```python
from build123d import *

# Parameters (mm, degrees)
SKETCH_2_W           = 42
SKETCH_2_H           = 42
EXTRUDE_1_DEPTH      = 69
SKETCH_3_R           = 12.5
EXTRUDE_2_DEPTH      = 2
SKETCH_4_R           = 4.5
EXTRUDE_3_DEPTH      = 1
SKETCH_5_R           = 4
EXTRUDE_4_DEPTH      = 18
EXTRUDE_5_DEPTH      = 1.5
EXTRUDE_5_DEPTH_BACK = 4
SKETCH_7_R           = 1.75
CUT_EXTRUDE_1_DEPTH  = 71.5


with BuildPart() as part:
    # 草图2 → 凸台-拉伸1 (new body)
    with BuildSketch(Plane(origin=(0, 0, 0), x_dir=(1, 0, 0), z_dir=(0, 1, 0))):
        with Locations((21, 21)):
            Rectangle(SKETCH_2_W, SKETCH_2_H)
    extrude(amount=EXTRUDE_1_DEPTH)

    # 草图3 → 凸台-拉伸2 (add)
    with BuildSketch(Plane(origin=(0, 69, 0), x_dir=(1, 0, 0), z_dir=(0, 1, 0))):
        with Locations(Location((21, 21, 0), (0, 0, 270))):
            Circle(SKETCH_3_R)
    extrude(amount=EXTRUDE_2_DEPTH)

    # 草图4 → 凸台-拉伸3 (add)
    with BuildSketch(Plane(origin=(0, 71, 0), x_dir=(1, 0, 0), z_dir=(0, 1, 0))):
        with Locations(Location((21, 21, 0), (0, 0, 270))):
            Circle(SKETCH_4_R)
    extrude(amount=EXTRUDE_3_DEPTH)

    # 草图5 → 凸台-拉伸4 (add)
    with BuildSketch(Plane(origin=(0, 72, 0), x_dir=(1, 0, 0), z_dir=(0, 1, 0))):
        with Locations(Location((21, 21, 0), (0, 0, 270))):
            Circle(SKETCH_5_R)
    extrude(amount=EXTRUDE_4_DEPTH)

    # 草图6 → 凸台-拉伸5 (add, two sides: drawn at the far end of the back side and taken through both)
    with BuildSketch(Plane.XY.offset(-17).offset(-EXTRUDE_5_DEPTH_BACK)):
        with BuildLine():
            Line((22.254851431, 87), (22.254851431, 76))
            ThreePointArc((22.254851431, 76), (21, 74.745148569), (19.745148569, 76))
            Line((19.745148569, 76), (19.745148569, 87))
            ThreePointArc((19.745148569, 87), (21, 88.254851431), (22.254851431, 87))
        make_face()
    extrude(amount=EXTRUDE_5_DEPTH + EXTRUDE_5_DEPTH_BACK)

    # 草图7 → 切除-拉伸1 (cut)
    with BuildSketch(Plane(origin=(0, 69, 0), x_dir=(1, 0, 0), z_dir=(0, 1, 0))):
        with Locations(Location((5.5, 36.5, 0), (0, 0, 270))):
            Circle(SKETCH_7_R)
        with Locations(Location((36.5, 36.5, 0), (0, 0, 90))):
            Circle(SKETCH_7_R)
        with Locations(Location((36.5, 5.5, 0), (0, 0, 270))):
            Circle(SKETCH_7_R)
        with Locations(Location((5.5, 5.5, 0), (0, 0, 90))):
            Circle(SKETCH_7_R)
    extrude(amount=-CUT_EXTRUDE_1_DEPTH, mode=Mode.SUBTRACT)


solid = part.part
```
Verification items for the finished model (mm, model axes). A direction names the side the tool comes from. Round coordinates to 2 decimals unless told otherwise and drop trailing zeros. Order: outer loops, then holes, each group sorted by start corner. A loop starts at its lowest first (then second) coordinate and runs counter-clockwise, first axis right, second up. Notation, with made-up numbers: (-12, 62.5) - (45, 62.5) arc R5 cw to (45, 66.5) - close; hole circle Ø11 at (53.5, 85). An arc over 180 degrees is marked (long way). Use CSV: the item, a comma, the result in double quotes. Start each with the question number.
1) Section check B-B, the plane z = -5.5. Record the cut outline in (x, y).
2) Mould release check, pull along Z, two halves, no side actions. Record for faces 1 (the flat face through (19.745, 81, -16)), 2 (the cylindrical face through (13.394, 69.986, -30.92)), 3 (the cylindrical face through (38.21, 34.98, -36.12)): +Z half, -Z half, draft (parallel to the pull), parting line (faces both ways), or undercut.
3) Access from +Z, -Z, +X, -X, +Y, -Y to the whole of each face (thin tool, end or side, straight path). Record for faces 4 (the flat face through (30, 69, -12)), 5 (the cylindrical face through (21.028, 74.745, -16.363)), 6 (the cylindrical face through (20.972, 88.255, -16.363)), 7 (the flat face through (22.255, 82, -16)), 8 (the flat face through (21, 82, -15.5)).
4) Section check A-A, the plane x = 36.5. Record the cut outline in (y, z).
5) Go/stop test with flat-tipped pins: P1, Ø0.9, axis at y = 82, z = -16.5, coming from the -X side; P2, Ø0.8, axis at x = 21.5, y = 80, coming from the +Z side; P3, Ø4, axis at x = 17, z = -32, coming from the +Y side. Record where each tip stops, or that it passes through.
6) Section check C-C, the plane y = 43.5. Record the cut outline in (x, z).
7) Thickness scan on L1, parallel to X at y = 26.5, z = -5.5; L2, parallel to Z at x = 6.5, y = 33; L3, parallel to Y at x = 25.5, z = -27. Record the ranges inside material, lowest first.
8) Section check D-D, the plane x = 21. Record the cut outline in (y, z), plus the area to 3 significant figures.
Answers:
1,outline,"(0, 0) - (3.75, 0) - (3.75, 69) - (0, 69) - close; (7.25, 0) - (34.75, 0) - (34.75, 69) - (7.25, 69) - close; (38.25, 0) - (42, 0) - (42, 69) - (38.25, 69) - close"
2,face 1,"draft"
2,face 2,"parting line"
2,face 3,"undercut"
3,face 4,"+Y"
3,face 5,"+Z"
3,face 6,"+Z, +Y"
3,face 7,"+Z, +X, +Y"
3,face 8,"+Z, +X, -X, +Y"
4,outline,"(0, -42) - (69, -42) - (69, -38.25) - (0, -38.25) - close; (0, -34.75) - (69, -34.75) - (69, -7.25) - (0, -7.25) - close; (0, -3.75) - (69, -3.75) - (69, 0) - (0, 0) - close"
5,P1,"stops at x = 19.75"
5,P2,"stops at z = -15.5"
5,P3,"stops at y = 71"
6,outline,"(0, -42) - (42, -42) - (42, 0) - (0, 0) - close; hole circle Ø3.5 at (5.5, -36.5); hole circle Ø3.5 at (5.5, -5.5); hole circle Ø3.5 at (36.5, -36.5); hole circle Ø3.5 at (36.5, -5.5)"
7,L1,"x = 0 to 3.75, 7.25 to 34.75, 38.25 to 42"
7,L2,"z = -42 to -37.94, -35.06 to -6.94, -4.06 to 0"
7,L3,"y = 0 to 71"
8,outline,"(0, -42) - (69, -42) - (69, -33.5) - (71, -33.5) - (71, -25.5) - (72, -25.5) - (72, -25) - (90, -25) - (90, -17) - (88.25, -17) - (88.25, -15.5) - (74.75, -15.5) - (74.75, -17) - (72, -17) - (72, -16.5) - (71, -16.5) - (71, -8.5) - (69, -8.5) - (69, 0) - (0, 0) - close"
8,area,"3,120 mm²"
